The figure shows three views and two pictorial views of one solid part (mm, origin at its lowest corner). Answer the questions. Give positions to 0.01 mm unless a question says otherwise; leave off trailing zeros. Loops run counter-clockwise (first coordinate to the right, second up) from the corner with the lowest first, then second, coordinate; pieces in that order, holes last. Notation, with made-up numbers: M 26.5,42.5 L 36.5,42.5 A6 cw 36.5,47.5 Z; hole C 69.5,-14 d3. An arc over 180 degrees is marked long. Write item = value, one per line. Start each with the question number.
1. Consider L1, parallel to Y at x = 14.5, z = 1.65; L2, parallel to X at y = 2.5, z = 2.65; L3, parallel to X at y = 2.75, z = 0.45. Determine where each line is inside the solid, lowest interval first. Write a range as [from, to].
2. Section A-A on x = 63.5 is taken. Determine the outline of the cut face in (y, z).
3. Section C-C on y = 4.5 is taken. Determine the outline of the cut face in (x, z), plus the area to 3 significant figures.
4. Section B-B on z = 1.35 is taken. Give the number of separate pieces and of enclosed holes in the cut face, plus the area to 3 significant figures.
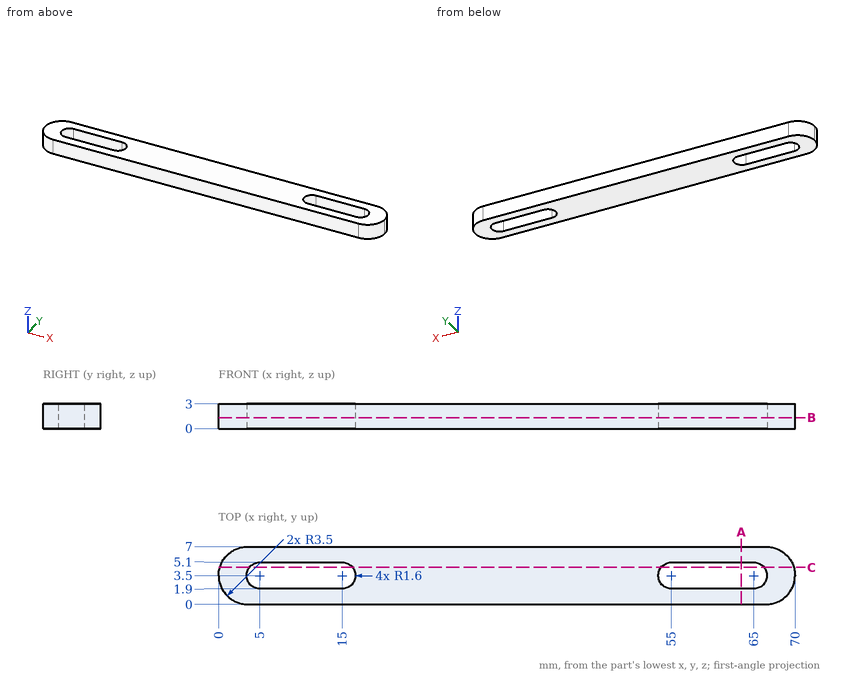
Verdict:
q1.L1 = [0, 1.9], [5.1, 7]
q1.L2 = [0.15, 3.75], [16.25, 53.75], [66.25, 69.85]
q1.L3 = [0.08, 3.59], [16.41, 53.59], [66.41, 69.92]
q2.outline = M 0,0 L 1.9,0 L 1.9,3 L 0,3 Z; M 5.1,0 L 7,0 L 7,3 L 5.1,3 Z
q3.outline = M 0.15,0 L 3.75,0 L 3.75,3 L 0.15,3 Z; M 16.25,0 L 53.75,0 L 53.75,3 L 16.25,3 Z; M 66.25,0 L 69.85,0 L 69.85,3 L 66.25,3 Z
q3.area = 134 mm2
q4.separate_pieces = 1
q4.enclosed_holes = 2
q4.area = 399 mm2
